Geometry: see drawing. Coordinates: mm, zero at the bounding-box minimum. Give positions to 0.01 mm unless a question says otherwise; leave off trailing zeros. Loops run counter-clockwise (first coordinate to the right, second up) from the corner with the lowest first, then second, coordinate; pieces in that order, holes last. Notation, with made-up numbers: M 3.25,7 L 37.25,7 A12 cw 37.25,19 Z; hole C 20.5,13.25 d9. An arc over 180 degrees is marked long. Put each result on its own line as item: value.
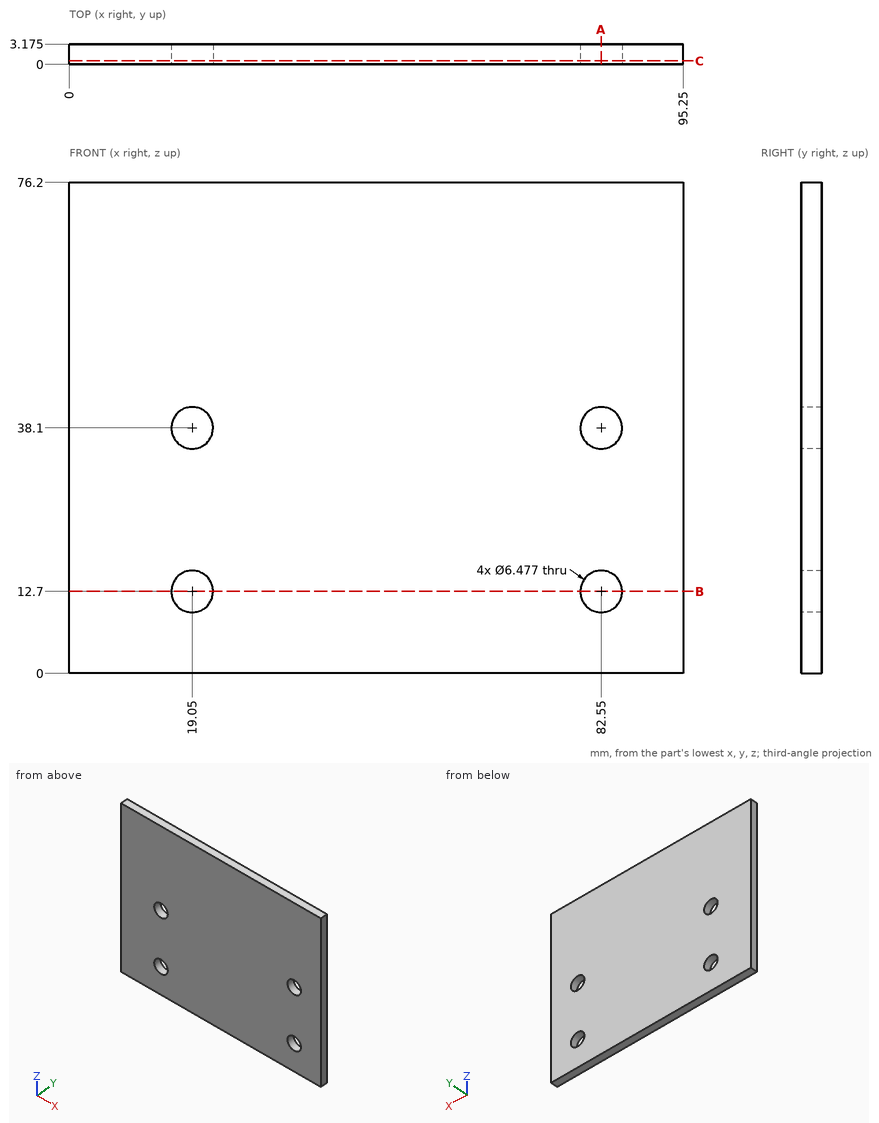
Item 1: Line query: probe 1 along X at (y, z) = (1.75, 38.1); probe 2 along Z at (x, y) = (19.05, 2.1); probe 3 along X at (y, z) = (2.55, 36). Output: solid intervals per line, ascending. Write a range as [from, to].
Output values:
probe 1: [0, 15.81], [22.29, 79.31], [85.79, 95.25]
probe 2: [0, 9.46], [15.94, 34.86], [41.34, 76.2]
probe 3: [0, 16.58], [21.52, 80.08], [85.02, 95.25]
Item 2: Section B-B on z = 12.7. Count the separate pieces of the cut face and the enclosed holes in it, then the cut area to 3 significant figures.
Output values:
separate pieces: 3
enclosed holes: 0
area: 261 mm²
Item 3: Section C-C on y = 0.55. Output: boundary loops of the cut face in (x, z).
Output values:
outline: M 0,0 L 95.25,0 L 95.25,76.2 L 0,76.2 Z; hole C 19.05,12.7 d6.48; hole C 19.05,38.1 d6.48; hole C 82.55,12.7 d6.48; hole C 82.55,38.1 d6.48
Item 4: Section A-A on x = 82.55. Output: boundary loops of the cut face in (y, z) (1 decimal).
Output values:
outline: M 0,0 L 3.2,0 L 3.2,9.5 L 0,9.5 Z; M 0,15.9 L 3.2,15.9 L 3.2,34.9 L 0,34.9 Z; M 0,41.3 L 3.2,41.3 L 3.2,76.2 L 0,76.2 Z
Item 5: Pin query (flat end, axial travel): pin 1 Ø10.5 at (x, z) = (19.05, 38.1) entering from -Y. Return the tip coordinate at first contact, or that it passes through.
Output values:
pin 1: y = 0
